CAD build for the part. Positions are in the model's coordinates, mm. A direction names the side the tool comes from. Coordinates: 2 decimals unless noted, no trailing zeros. Loops run counter-clockwise (first coordinate to the right, second up) from the corner with the lowest first, then second, coordinate; pieces in that order, holes last. Notation, with made-up numbers: (48.5, 78) -> (60.5, 78) arc R14 cw to (60.5, 99) -> close; hole circle Ø1 at (17, 53.5). An arc over 180 degrees is marked (long way). Return JSON: item names as keys, results as strings. Group by question number.
(1) Probe L1, parallel to X at y = -1.5, z = 6.75; L2, parallel to X at y = 7, z = 16.75; L3, parallel to Y at x = 240, z = 3. List the from-to ranges inside material, lowest first.
(2) Tool access for faces 1 (the face through (236, 4.588, 9)), 2 (the face through (-70.376, -4, 9)), 3 (the face through (393.624, -4, 9)), 4 (the face through (-80, -75.412, 9)), 5 (the face through (404, -75.412, 9)): list every direction of +Z, -Z, +X, -X, +Y, -Y with a clear straight run to the whole face (end or side of a thin tool).
(3) Saw through at B-B on y = 13. Write the cut outline in (x, z).
(4) Mould opens along X. For faces 6 (the face through (256, 22.588, 9)), 7 (the face through (237, -13.412, 9)), 8 (the face through (17.624, 15, 9)) say: pulls with the +X half, pulls with the -X half, needs draft (parallel to the pull), parting line crosses it, or undercut.
(5) Saw through at C-C on x = 191.5. Write the cut outline in (y, z).
(6) Saw through at D-D on x = 342. Write the cut outline in (y, z), then the cut area to 3 significant figures.
(7) Flat gauge pins, fed straight in: pin 1 Ø5.5 at (y, z) = (-89.5, 9.5) entering from +X; pin 2 Ø8 at (y, z) = (17.5, 8) entering from +X; pin 3 Ø6.5 at (y, z) = (-4, 12) entering from -X. Where does each tip first touch, or does it go through?
(8) Saw through at A-A on x = 247.5. Write the cut outline in (y, z), then the cut area to 3 significant figures.
Autodesk Inventor part; units mm, degrees
ref_plane "YZ Plane" through (0, 0, 0) normal (1, 0, 0) x (0, 1, 0)
ref_plane "XZ Plane" through (0, 0, 0) normal (0, 1, 0) x (-1, 0, 0)
ref_plane "XY Plane" through (0, 0, 0) normal (0, 0, 1) x (1, 0, 0)
sketch "Sketch1" plane through (0, 0, 0) normal (0, 0, 1) x (1, 0, 0)
  line L0 (393.6245, -95.4118) -> (-70.3755, -95.4118)
  line L1 (17.6245, 22.5882) -> (117.6245, 22.5882)
  line L2 (117.6245, 22.5882) -> (117.6245, 4.5882)
  line L3 (17.6245, 4.5882) -> (17.6245, 22.5882)
  line L4 (-70.3755, 4.5882) -> (17.6245, 4.5882)
  line L5 (305.6245, 22.5882) -> (205.6245, 22.5882)
  line L6 (205.6245, 22.5882) -> (205.6245, 4.5882)
  line L7 (305.6245, 4.5882) -> (305.6245, 22.5882)
  line L8 (117.6245, 4.5882) -> (205.6245, 4.5882)
  line L9 (305.6245, 4.5882) -> (393.6245, 4.5882)
  line L10 (-88.3755, -15.4118) -> (-70.3755, -15.4118)
  line L11 (-70.3755, -75.4118) -> (-88.3755, -75.4118)
  line L12 (-88.3755, -75.4118) -> (-88.3755, -15.4118)
  line L13 (-70.3755, -95.4118) -> (-70.3755, -75.4118)
  line L14 (-70.3755, -15.4118) -> (-70.3755, 4.5882)
  line L15 (393.6245, -15.4118) -> (411.6245, -15.4118)
  line L16 (411.6245, -15.4118) -> (411.6245, -75.4118)
  line L17 (411.6245, -75.4118) -> (393.6245, -75.4118)
  line L18 (393.6245, 4.5882) -> (393.6245, -15.4118)
  line L19 (393.6245, -75.4118) -> (393.6245, -95.4118)
  point P0 (0, 0)
  dimension "d0" = 464
  dimension "d4" = 100
  dimension "d5" = 18
  dimension "d9" = 100
  dimension "d10" = 18
  dimension "d13" = 18
  dimension "d14" = 60
  dimension "d17" = 20
  dimension "d19" = 60
  dimension "d20" = 18
  dimension "d21" = 100
  dimension "d37" = 88
  dimension "d38" = 88
  dimension "d39" = 88
extrude "Extrusion1" add sketch "Sketch1" along normal blind 18
sketch "Sketch2" plane through (0, 0, 18) normal (0, 0, 1) x (1, 0, 0)
  line L0 (-70.3755, -15.4118) -> (-71.5069, -14.2805)
  line L1 (-70.3755, -15.4118) -> (-68.7755, -15.4118) construction
  line L2 (-70.3755, -75.4118) -> (-71.5069, -76.5432)
  line L3 (17.6245, 4.5882) -> (16.4931, 5.7195)
  line L4 (17.6245, 4.5882) -> (19.2245, 4.5882) construction
  line L5 (117.6245, 4.5882) -> (118.7558, 5.7195)
  line L6 (205.6245, 4.5882) -> (204.4931, 5.7195)
  line L7 (305.6245, 4.5882) -> (306.7558, 5.7195)
  line L8 (393.6245, -15.4118) -> (394.7558, -14.2805)
  line L9 (393.6245, -75.4118) -> (394.7558, -76.5432)
  circle A0 centre (-71.5069, -14.2805) radius 1.6
  circle A1 centre (-71.5069, -76.5432) radius 1.6
  circle A2 centre (16.4931, 5.7195) radius 1.6
  circle A3 centre (118.7558, 5.7195) radius 1.6
  circle A4 centre (204.4931, 5.7195) radius 1.6
  circle A5 centre (306.7558, 5.7195) radius 1.6
  circle A6 centre (394.7558, -14.2805) radius 1.6
  circle A7 centre (394.7558, -76.5432) radius 1.6
  point P0 (0, 0)
  dimension "d22" = 1.6
  dimension "d23" = 135
  dimension "d24" = 1.6
  dimension "d25" = 135
  dimension "d26" = 3.2
  dimension "d27" = 3.2
  dimension "d28" = 3.2
  dimension "d29" = 3.2
  dimension "d30" = 3.2
  dimension "d32" = 3.2
  dimension "d33" = 3.2
  dimension "d34" = 3.2
extrude "Extrusion2" cut sketch "Sketch2" against normal blind 20
sketch "Sketch3" plane through (0, 0, 18) normal (0, 0, 1) x (1, 0, 0)
  line L0 (211.3165, 4.5882) -> (261.3165, 4.5882)
  line L1 (261.3165, 4.5882) -> (261.3165, -13.4118)
  line L2 (261.3165, -13.4118) -> (211.3165, -13.4118)
  line L3 (211.3165, -13.4118) -> (211.3165, 4.5882)
  line L4 (305.6245, 22.5882) -> (205.6245, 22.5882)
  line L5 (205.6245, 22.5882) -> (205.6245, 6.8509)
  line L6 (328.7435, 4.5882) -> (378.7435, 4.5882)
  line L7 (378.7435, 4.5882) -> (378.7435, -13.4118)
  line L8 (378.7435, -13.4118) -> (328.7435, -13.4118)
  line L9 (328.7435, -13.4118) -> (328.7435, 4.5882)
  line L10 (393.6245, 4.5882) -> (307.8872, 4.5882)
  point P0 (0, 0)
  dimension "d40" = 50
  dimension "d41" = 18
  dimension "d42" = 18
  dimension "d43" = 5.692
  dimension "d44" = 50
  dimension "d45" = 18
  dimension "d46" = 67.427
  dimension "d47" = 0
extrude "Extrusion3" cut sketch "Sketch3" against normal blind 18
sketch "Sketch4" plane through (0, 0, 18) normal (0, 0, 1) x (1, 0, 0)
  line L0 (211.3165, 4.5882) -> (212.4478, 3.4568)
  line L1 (211.3165, 4.5882) -> (212.9165, 4.5882) construction
  line L2 (211.3165, -13.4118) -> (212.4478, -12.2805)
  line L3 (211.3165, -13.4118) -> (212.9165, -13.4118) construction
  line L4 (261.3165, -13.4118) -> (260.1851, -12.2805)
  line L5 (261.3165, 4.5882) -> (260.1851, 3.4568)
  circle A0 centre (212.4478, 3.4568) radius 1.6
  circle A1 centre (212.4478, -12.2805) radius 1.6
  circle A2 centre (260.1851, 3.4568) radius 1.6
  circle A3 centre (260.1851, -12.2805) radius 1.6
  line L6 (328.7435, -13.4118) -> (329.8748, -12.2805)
  line L7 (328.7435, -13.4118) -> (330.3435, -13.4118) construction
  line L8 (378.7435, -13.4118) -> (377.6121, -12.2805)
  circle A4 centre (377.6121, -12.2805) radius 1.6
  circle A5 centre (329.8748, -12.2805) radius 1.6
  point P0 (0, 0)
  dimension "d50" = 1.6
  dimension "d51" = 45
  dimension "d52" = 1.6
  dimension "d53" = 45
  dimension "d54" = 3.2
  dimension "d55" = 3.2
  dimension "d56" = 3.2
  dimension "d57" = 3.2
  dimension "d58" = 1.6
  dimension "d59" = 45
  dimension "d60" = 3.2
  dimension "d61" = 3.2
extrude "Extrusion4" cut sketch "Sketch4" against normal blind 20
properties part number "laterales" material "Wood (Birch)"
Geometry results:
{
 "1": {"L1": "-70.38 to 211.32, 261.32 to 328.74, 378.74 to 393.62", "L2": "17.62 to 117.62, 205.62 to 305.62", "L3": "-95.41 to -13.41, 4.59 to 22.59"},
 "2": {"face 1": "+Z, -Z", "face 2": "+Z, -Z, -X, +Y", "face 3": "+Z, -Z, +X, +Y", "face 4": "+Z, -Z, -X, -Y", "face 5": "+Z, -Z, +X, -Y"},
 "3": {"outline": "(17.62, 0) -> (117.62, 0) -> (117.62, 18) -> (17.62, 18) -> close; (205.62, 0) -> (305.62, 0) -> (305.62, 18) -> (205.62, 18) -> close"},
 "4": {"face 6": "needs draft", "face 7": "undercut", "face 8": "pulls with the -X half"},
 "5": {"outline": "(-95.41, 0) -> (4.59, 0) -> (4.59, 18) -> (-95.41, 18) -> close"},
 "6": {"outline": "(-95.41, 0) -> (-13.41, 0) -> (-13.41, 18) -> (-95.41, 18) -> close", "area": "1,480 mm²"},
 "7": {"pin 1": "x = 393.62", "pin 2": "x = 305.62", "pin 3": "x = -70.38"},
 "8": {"outline": "(-95.41, 0) -> (-13.41, 0) -> (-13.41, 18) -> (-95.41, 18) -> close; (4.59, 0) -> (22.59, 0) -> (22.59, 18) -> (4.59, 18) -> close", "area": "1,800 mm²"}
}
